Can you work these out from the drawing? Everything is in mm from the part's minimum corner. A direction names the side the tool comes from. Give positions to 0.01 mm unless a question says otherwise; leave off trailing zeros. Loops run counter-clockwise (first coordinate to the right, second up) from the corner with the lowest first, then second, coordinate; pieces in that order, holes last. Notation, with made-up numbers: (51, 43.25) -> (99, 43.25) arc R29 cw to (99, 71.25) -> close; hole circle Ø11 at (75, 37.25). An arc over 180 degrees is marked (long way). Return JSON: item names as keys, results as strings. Group by question number.
Q1. I need wall thicknesses on line 1 along Z through (x, y) = (6.25, 4); line 2 along Y through (x, z) = (6.3, 38.5); line 3 along Y through (x, z) = (2.55, 20). Which ranges of each line are inside material? Lowest first, please. Write a range as [from, to].
Q2. Suppose I cut it at C-C, the plane x = 7.5. Please give me the cut outline in (y, z).
Q3. Suppose I cut it at A-A, the plane y = 4. Please give me the cut outline in (x, z), and give its area (3 significant figures).
Q4. Which directions (+Z, -Z, +X, -X, +Y, -Y) give clear straight access to the entire face, cutting with the end or side of a thin tool? Please do the marked faces 1, 2, 3, 4 and 5.
Q5. Will these pins go through, and if not, where does the flat tip stop? pin 1 (3 mm diameter, centred on y = 4, z = 73, fed in from -X); pin 2 (3 mm diameter, centred on x = 3.5, y = 56, fed in from -Z); pin 3 (17 mm diameter, centred on y = 54, z = 41.5, fed in from -X); pin 4 (3 mm diameter, centred on x = 6.5, y = 49, fed in from +Z).
Q6. Suppose I cut it at D-D, the plane x = 1.25. Please give me the cut outline in (y, z), and give its area (3 significant figures).
Q7. Suppose I cut it at B-B, the plane z = 38.5. Please give me the cut outline in (x, y).
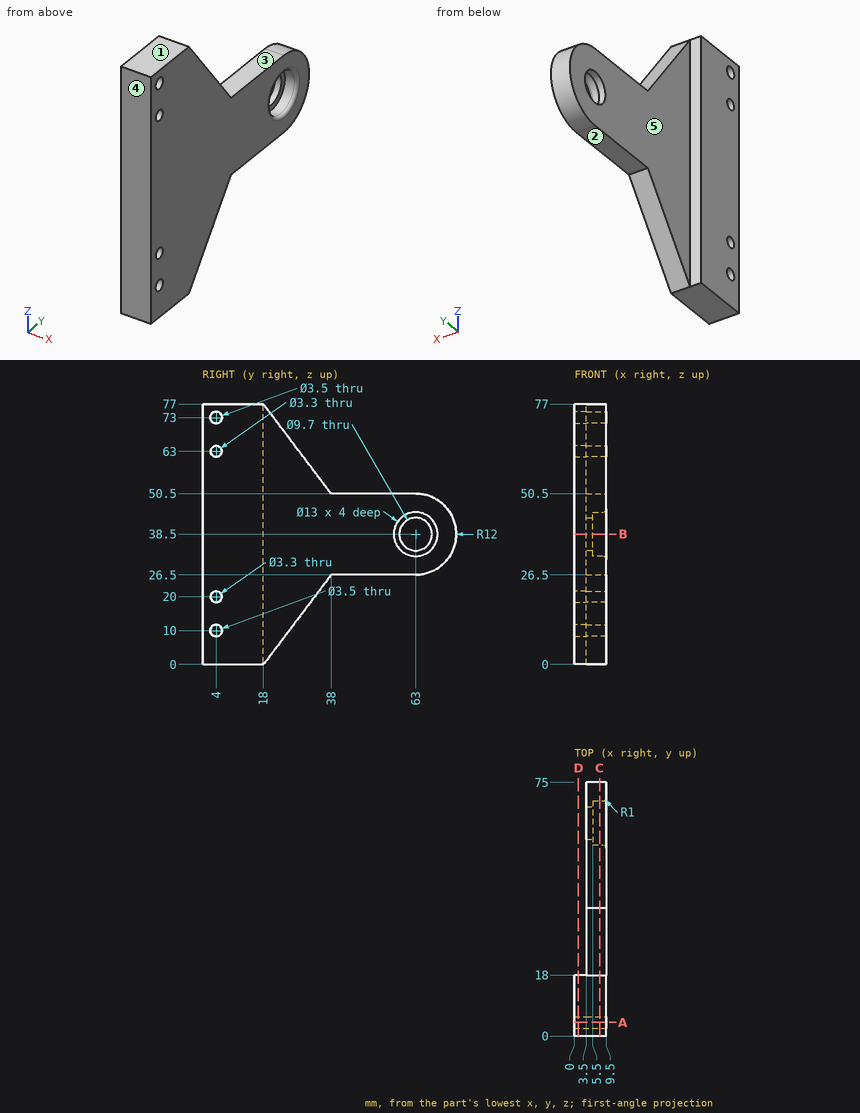
Ans:
{
 "1": {"line 1": "z = [0, 8.25], [11.75, 18.35], [21.65, 61.35], [64.65, 71.25], [74.75, 77]", "line 2": "y = [0, 56.5], [69.5, 75]", "line 3": "y = [0, 2.35], [5.65, 18]"},
 "2": {"outline": "(0, 0) -> (18, 0) -> (38, 26.5) -> (63, 26.5) arc R12 ccw to (63, 50.5) -> (38, 50.5) -> (18, 77) -> (0, 77) -> close; hole circle Ø3.5 at (4, 10); hole circle Ø3.5 at (4, 73); hole circle Ø3.3 at (4, 20); hole circle Ø3.3 at (4, 63); hole circle Ø13 at (63, 38.5)"},
 "3": {"outline": "(0, 0) -> (9.5, 0) -> (9.5, 8.25) -> (0, 8.25) -> close; (0, 11.75) -> (9.5, 11.75) -> (9.5, 18.35) -> (0, 18.35) -> close; (0, 21.65) -> (9.5, 21.65) -> (9.5, 61.35) -> (0, 61.35) -> close; (0, 64.65) -> (9.5, 64.65) -> (9.5, 71.25) -> (0, 71.25) -> close; (0, 74.75) -> (9.5, 74.75) -> (9.5, 77) -> (0, 77) -> close", "area": "602 mm^2"},
 "4": {"face 1": "+Z, +X, -X, +Y, -Y", "face 2": "-Z, +X, -X, +Y", "face 3": "+Z, +X, -X, +Y", "face 4": "+Z, -Z, +X, -X, -Y", "face 5": "+Z, -Z, -X, +Y"},
 "5": {"pin 1": "passes through", "pin 2": "stops at z = 26.5", "pin 3": "stops at x = 3.5", "pin 4": "stops at z = 50.5"},
 "6": {"outline": "(0, 0) -> (18, 0) -> (18, 77) -> (0, 77) -> close; hole circle Ø3.5 at (4, 10); hole circle Ø3.5 at (4, 73); hole circle Ø3.3 at (4, 20); hole circle Ø3.3 at (4, 63)", "area": "1,350 mm^2"},
 "7": {"outline": "(0, 0) -> (9.5, 0) -> (9.5, 55.5) arc R1 ccw to (8.5, 56.5) -> (5.5, 56.5) -> (5.5, 58.15) -> (3.5, 58.15) -> (3.5, 18) -> (0, 18) -> close; (3.5, 67.85) -> (5.5, 67.85) -> (5.5, 69.5) -> (8.5, 69.5) arc R1 ccw to (9.5, 70.5) -> (9.5, 75) -> (3.5, 75) -> close"}
}
